```python
from build123d import *

# Parameters (mm, degrees)
SKETCH1_R               = 69
BOSS_EXTRUDE1_DEPTH     = 30
SKETCH2_W               = 125
SKETCH2_H               = 125
BOSS_EXTRUDE2_DEPTH     = 3
SKETCH3_R               = 2.75
CUT_EXTRUDE1_DEPTH      = 3
SKETCH4_R               = 66
CUT_EXTRUDE2_DEPTH      = 103.088197163
FILLET1_R               = 10
CUT_EXTRUDE3_DEPTH      = 103.088197163
BOSS_EXTRUDE4_DEPTH     = 30
CIRPATTERN2_COUNT       = 4
BOSS_EXTRUDE5_DEPTH     = 30
CUT_EXTRUDE4_DEPTH      = 12
CUT_EXTRUDE4_DEPTH_BACK = 12
SKETCH10_R              = 66
SKETCH11_R              = 15
BOSS_EXTRUDE6_DEPTH     = 30
SKETCH12_R              = 1.75
BOSS_EXTRUDE9_DEPTH     = 30
CUT_EXTRUDE5_START      = -25
SKETCH12_3_R            = 1.75
CUT_EXTRUDE5_DEPTH      = 5
SKETCH14_R              = 12
CUT_EXTRUDE6_DEPTH      = 103.088197329


with BuildPart() as part:
    # Sketch1 → Boss-Extrude1 (new body)
    with BuildSketch(Plane(origin=(0, 0, 0), x_dir=(1, 0, 0), z_dir=(0, 1, 0))):
        with Locations(Location((0, 0, 0), (0, 0, 270))):
            Circle(SKETCH1_R)
    extrude(amount=BOSS_EXTRUDE1_DEPTH)

    # Sketch2 → Boss-Extrude2 (add)
    with BuildSketch(Plane(origin=(0, 30, 0), x_dir=(1, 0, 0), z_dir=(0, 1, 0))):
        Rectangle(SKETCH2_W, SKETCH2_H)
    extrude(amount=-BOSS_EXTRUDE2_DEPTH)

    # Sketch3 → Cut-Extrude1 (cut)
    with BuildSketch(Plane(origin=(0, 30, 0), x_dir=(1, 0, 0), z_dir=(0, 1, 0))):
        with Locations(Location((55, 55, 0), (0, 0, 270))):
            Circle(SKETCH3_R)
        with Locations(Location((-55, 55, 0), (0, 0, 270))):
            Circle(SKETCH3_R)
        with Locations(Location((-55, -55, 0), (0, 0, 270))):
            Circle(SKETCH3_R)
        with Locations(Location((55, -55, 0), (0, 0, 270))):
            Circle(SKETCH3_R)
    extrude(amount=-CUT_EXTRUDE1_DEPTH, mode=Mode.SUBTRACT)

    # Sketch4 → Cut-Extrude2 (cut, through all)
    with BuildSketch(Plane.XZ):
        with Locations(Location((0, 0, 0), (0, 0, 270))):
            Circle(SKETCH4_R)
    extrude(amount=-CUT_EXTRUDE2_DEPTH, mode=Mode.SUBTRACT)

    # Fillet1
    fillet1_edges = [part.edges().sort_by_distance(p)[0] for p in [
        (-62.5, 28.5, 62.5),
        (-62.5, 28.5, -62.5),
        (62.5, 28.5, -62.5),
        (62.5, 28.5, 62.5),
    ]]
    fillet(fillet1_edges, radius=FILLET1_R)

    # Sketch6 → Cut-Extrude3 (cut, through all)
    with BuildSketch(Plane(origin=(0, 0, 0), x_dir=(0, 0, -1), z_dir=(1, 0, 0))):
        with BuildLine():
            Line((-8, 0), (-8, 12))
            ThreePointArc((-8, 12), (0, 20), (8, 12))
            Line((8, 12), (8, 0))
            ThreePointArc((8, 0), (0, -8), (-8, 0))
        make_face()
    extrude(amount=CUT_EXTRUDE3_DEPTH, mode=Mode.SUBTRACT)

    # Sketch8 → Boss-Extrude4 (add)
    with BuildSketch(Plane(origin=(0, 30, 0), x_dir=(1, 0, 0), z_dir=(0, 1, 0))):
        Polygon((41.790010768, 54.659354186), (33.870414819, 46.739758236), (46.739758236, 33.870414819), (54.659354186, 41.790010768), align=None)
        Polygon((41.790010768, 50.416713499), (50.416713499, 41.790010768), (46.739758236, 38.113055506), (38.113055506, 46.739758236), align=None, mode=Mode.SUBTRACT)
    boss_extrude4 = extrude(amount=-BOSS_EXTRUDE4_DEPTH)

    # CirPattern2: Boss-Extrude4 ×4 about axis
    cirpattern2_axis = Axis((0, 0, 0), (0, 1, 0))
    for i in range(1, CIRPATTERN2_COUNT):
        add(boss_extrude4.rotate(cirpattern2_axis, i * 360 / CIRPATTERN2_COUNT))

    # Sketch9 → Boss-Extrude5 (add)
    with BuildSketch(Plane(origin=(0, 30, 0), x_dir=(1, 0, 0), z_dir=(0, 1, 0))):
        Polygon((46.739758236, 33.870414819), (33.870414819, 46.739758236), (0, 8), (-33.870414819, 46.739758236), (-46.739758236, 33.870414819), (-8, 0), (-46.739758236, -33.870414819), (-33.870414819, -46.739758236), (0, -8), (33.870414819, -46.739758236), (46.739758236, -33.870414819), (8, 0), align=None)
    extrude(amount=-BOSS_EXTRUDE5_DEPTH)

    # Sketch10 → Cut-Extrude4 (cut, two sides: drawn at the far end of the back side and taken through both)
    with BuildSketch(Plane(origin=(0, 15, 0), x_dir=(1, 0, 0), z_dir=(0, 1, 0)).offset(-CUT_EXTRUDE4_DEPTH_BACK)):
        with Locations(Location((0, 0, 0), (0, 0, 52.925119379))):
            Circle(SKETCH10_R)
    extrude(amount=CUT_EXTRUDE4_DEPTH + CUT_EXTRUDE4_DEPTH_BACK, mode=Mode.SUBTRACT)

    # Sketch11 → Boss-Extrude6 (add)
    with BuildSketch(Plane.XZ):
        with Locations(Location((0, 0, 0), (0, 0, 290.612180744))):
            Circle(SKETCH11_R)
    extrude(amount=-BOSS_EXTRUDE6_DEPTH)

    # Sketch12 → Boss-Extrude9 (add)
    with BuildSketch(Plane.XZ):
        with BuildLine():
            Line((5, 62.278453748), (5, 67.278453748))
            Line((5, 67.278453748), (-5, 67.278453748))
            Line((-5, 67.278453748), (-5, 62.278453748))
            ThreePointArc((-5, 62.278453748), (0, 57.278453748), (5, 62.278453748))
        make_face()
        with Locations(Location((0, 62.278453748, 0), (0, 0, 270))):
            Circle(SKETCH12_R, mode=Mode.SUBTRACT)
    boss_extrude9 = extrude(amount=-BOSS_EXTRUDE9_DEPTH)

    # Mirror1: Boss-Extrude9 across plane
    add(boss_extrude9.mirror(Plane.XY))

    # Sketch12<3> → Cut-Extrude5 (cut)
    with BuildSketch(Plane.XZ.offset(CUT_EXTRUDE5_START)):
        with BuildLine():
            Line((5, 62.278453748), (5, 67.278453748))
            Line((5, 67.278453748), (-5, 67.278453748))
            Line((-5, 67.278453748), (-5, 62.278453748))
            ThreePointArc((-5, 62.278453748), (0, 57.278453748), (5, 62.278453748))
        make_face()
        with Locations(Location((0, 62.278453748, 0), (0, 0, 270))):
            Circle(SKETCH12_3_R, mode=Mode.SUBTRACT)
    cut_extrude5 = extrude(amount=-CUT_EXTRUDE5_DEPTH, mode=Mode.SUBTRACT)

    # Mirror2: Cut-Extrude5 across plane
    add(cut_extrude5.mirror(Plane.XY), mode=Mode.SUBTRACT)

    # Sketch14 → Cut-Extrude6 (cut, through all)
    with BuildSketch(Plane(origin=(0, 30, 0), x_dir=(1, 0, 0), z_dir=(0, 1, 0))):
        with Locations(Location((0, 0, 0), (0, 0, 270))):
            Circle(SKETCH14_R)
    extrude(amount=-CUT_EXTRUDE6_DEPTH, mode=Mode.SUBTRACT)


solid = part.part
```
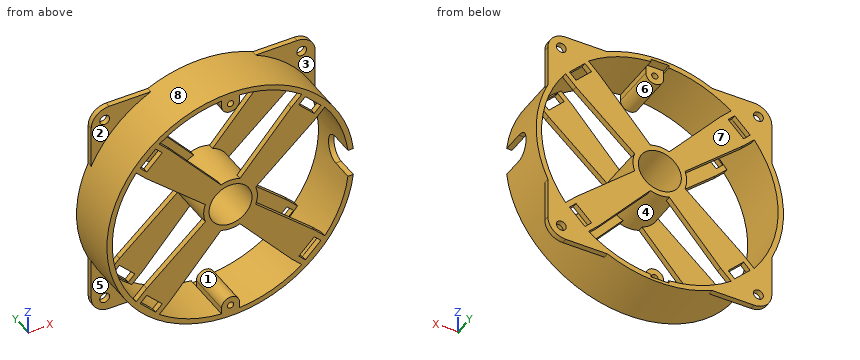
Geometry: final body of the model. Coordinates: model frame, mm. Face numbers are marked on the shaded views. A direction names the side the tool comes from. Round coordinates to 2 decimals unless told otherwise and drop trailing zeros. Loops run counter-clockwise (first coordinate to the right, second up) from the corner with the lowest first, then second, coordinate; pieces in that order, holes last.
Item 1: Mould query, pull axis Z, two halves, no side actions, for the marked faces 6, 7 and 8. Classes: released by +Z, released by -Z, zero draft, split by the parting line, or undercut.
Checked values:
face 6: undercut
face 7: zero draft
face 8: split by the parting line
Item 2: Line query: L1, parallel to X at y = 29.2, z = 55; L2, parallel to X at y = 18, z = 10; L3, parallel to Z at x = 5.5, y = 24.5. Output: solid intervals per line, ascending.
Checked values:
L1: x = -62.18 to -57.75, -52.25 to -36.48, 36.48 to 52.25, 57.75 to 62.18
L2: x = -68.27 to -65.24, -11.18 to -6.63, 6.63 to 11.18, 65.24 to 68.27
L3: z = -68.78 to -65.77, -13.96 to -10.67, 10.67 to 13.96, 65.77 to 68.78
Item 3: Reachability of the marked faces 1, 2, 3, 4 and 5 from +Z, -Z, +X, -X, +Y, -Y: full face, straight path, thin tool, end or side. Return the list, or none.
Checked values:
face 1: +Y, -Y
face 2: +Z, -X, -Y
face 3: +Z, +X, -Y
face 4: none
face 5: -Z, -X, -Y
Item 4: Section A-A, the plane y = 8.5. Output: boundary loops of the cut face in (x, z).
Checked values:
outline: circle Ø30 at (0, 0); (-5, -65.81) arc R66 cw to (-5, 65.81) - (-5, 62.28) arc R5 ccw to (5, 62.28) - (5, 65.81) arc R66 cw to (65.51, 8) - (68.53, 8) arc R69 ccw (long way) to (68.53, -8) - (65.51, -8) arc R66 cw to (5, -65.81) - (5, -62.28) arc R5 ccw to (-5, -62.28) - close; hole circle Ø24 at (0, 0); hole circle Ø3.5 at (0, -62.28); hole circle Ø3.5 at (0, 62.28)
Item 5: Section C-C, the plane z = 0. Output: boundary loops of the cut face in (x, y), plus the area to 3 significant figures.
Checked values:
outline: (-69, 0) - (-66, 0) - (-66, 30) - (-69, 30) - close; (-15, 0) - (-12, 0) - (-12, 30) - (-15, 30) - close; (12, 0) - (15, 0) - (15, 30) - (12, 30) - close; (66, 20) - (69, 20) - (69, 30) - (66, 30) - close
area: 300 mm2
Item 6: Section D-D, the plane z = 35.5. Output: boundary loops of the cut face in (x, y), plus the area to 3 significant figures.
Checked values:
outline: (-62.5, 27) - (-59.17, 27) - (-59.17, 0) - (-55.64, 0) - (-55.64, 30) - (-62.5, 30) - close; (-48.37, 0) - (-24.04, 0) - (-24.04, 3) - (-48.37, 3) - close; (-48.37, 27) - (-24.04, 27) - (-24.04, 30) - (-48.37, 30) - close; (24.04, 0) - (48.37, 0) - (48.37, 3) - (24.04, 3) - close; (24.04, 27) - (48.37, 27) - (48.37, 30) - (24.04, 30) - close; (55.64, 0) - (59.17, 0) - (59.17, 27) - (62.5, 27) - (62.5, 30) - (55.64, 30) - close
area: 524 mm2
Item 7: Contact query for flat-ended pins moving along their axis: P1, Ø4, axis at y = 13, z = 64, coming from the +X side; P2, Ø3, axis at y = 8.5, z = 20, coming from the +X side; P3, Ø0.9, axis at y = 28, z = -38.5, coming from the +X side. Output: stop coordinate, or through.
Checked values:
P1: stops at x = 30.28
P2: stops at x = 66.47
P3: stops at x = 62.5
Item 8: Section B-B, the plane x = 0. Output: boundary loops of the cut face in (y, z).
Checked values:
outline: (0, -69) - (30, -69) - (30, -67.28) - (25, -67.28) - (25, -64.03) - (0, -64.03) - close; (0, -60.53) - (25, -60.53) - (25, -57.28) - (0, -57.28) - close; (0, -15) - (30, -15) - (30, -12) - (0, -12) - close; (0, 12) - (30, 12) - (30, 15) - (0, 15) - close; (0, 57.28) - (25, 57.28) - (25, 60.53) - (0, 60.53) - close; (0, 64.03) - (25, 64.03) - (25, 67.28) - (30, 67.28) - (30, 69) - (0, 69) - close
